Study the drawing (mm; zero at the part's minimum x, y, z) and answer. A direction names the side the tool comes from. Round coordinates to 2 decimals unless told otherwise and drop trailing zeros. Write each loop counter-clockwise with the first axis right and the second up, starting at its lowest first coordinate (ties: lowest second). Pieces come first, ordered by that corner, then holes. Notation, with made-up numbers: (-35.75, 74) - (-18.75, 74) arc R30 ccw to (-18.75, 107) - close; hole circle Ø3 at (79, 56.25). An arc over 180 degrees is marked (long way). Return JSON: item names as keys, results as strings. Group by question number.
(1) Find the intervals of material crossed by line 1 along Z through (x, y) = (1.75, 16); line 2 along Y through (x, z) = (15, 25), in increasing order. Write a range as [from, to].
(2) Determine the mould class of the marked faces 3, 4 and 5 for opening direction Z: +Z half, -Z half, draft (parallel to the pull), parting line (faces both ways), or undercut.
(3) Section A-A, the plane y = 11 is taken. Write down the section's boundary in (x, z), then the cut area to 3 significant figures.
(4) Each of these flat-tipped pins is pushed along its axis until it touches: pin 1 (12 mm diameter, centred on x = 20, y = 9, fed in from +Z); pin 2 (1.4 mm diameter, centred on x = 24, z = 18, fed in from +Y). Where does it stop, or does it pass through?
(5) Section C-C, the plane z = 18 is taken. Write down the section's boundary in (x, y), then the cut area to 3 significant figures.
(6) Which of the six approach directions +Z, -Z, +X, -X, +Y, -Y give full straight-line access (tool end or side, diameter ignored) to the marked faces 1 and 2?
(7) Section D-D, the plane y = 29 is taken. Write down the section's boundary in (x, z), then the cut area to 3 significant figures.
(8) Section B-B, the plane x = 15 is taken. Write down the section's boundary in (y, z).
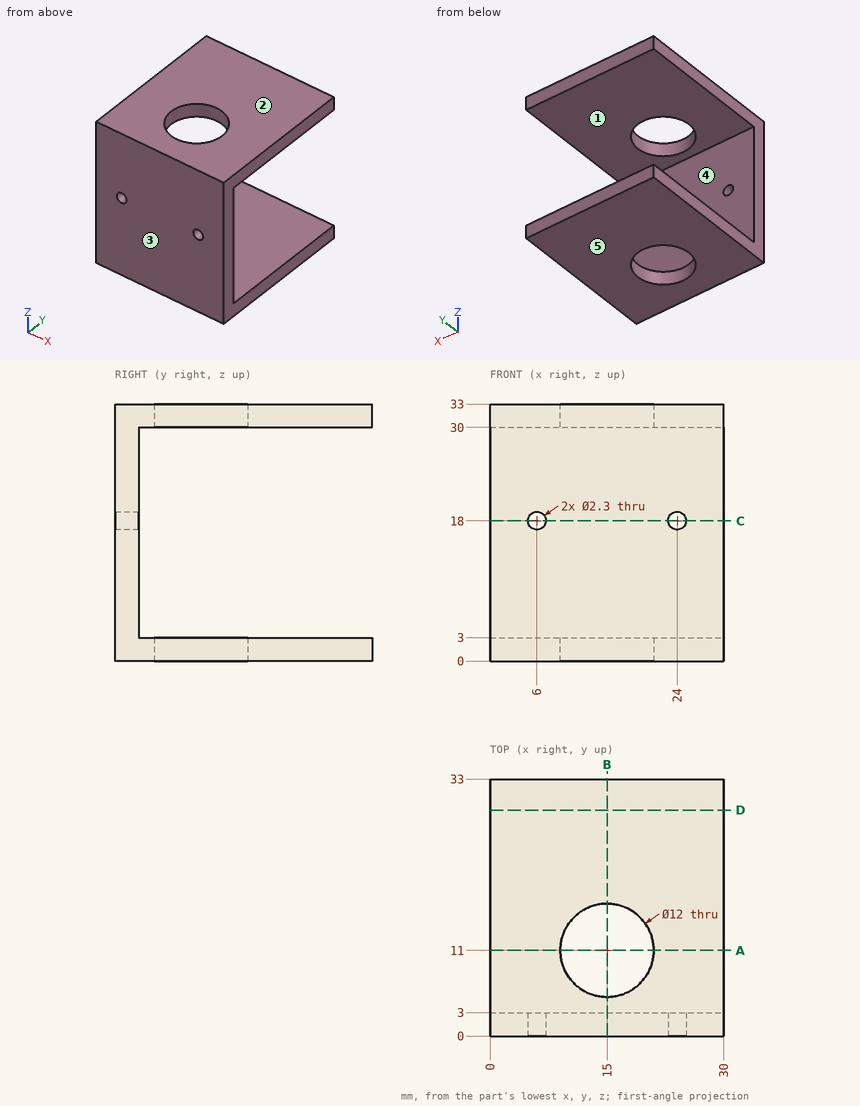
Working result:
{
 "1": {"line 1": "z = [0, 3], [30, 33]", "line 2": "y = [0, 3]"},
 "2": {"face 3": "draft", "face 4": "undercut", "face 5": "-Z half"},
 "3": {"outline": "(0, 0) - (9, 0) - (9, 3) - (0, 3) - close; (0, 30) - (9, 30) - (9, 33) - (0, 33) - close; (21, 0) - (30, 0) - (30, 3) - (21, 3) - close; (21, 30) - (30, 30) - (30, 33) - (21, 33) - close", "area": "108 mm^2"},
 "4": {"pin 1": "stops at z = 33", "pin 2": "passes through"},
 "5": {"outline": "(0, 0) - (4.85, 0) - (4.85, 3) - (0, 3) - close; (7.15, 0) - (22.85, 0) - (22.85, 3) - (7.15, 3) - close; (25.15, 0) - (30, 0) - (30, 3) - (25.15, 3) - close", "area": "76.2 mm^2"},
 "6": {"face 1": "+X, -X, +Y", "face 2": "+Z, +X, -X, +Y, -Y"},
 "7": {"outline": "(0, 0) - (30, 0) - (30, 3) - (0, 3) - close; (0, 30) - (30, 30) - (30, 33) - (0, 33) - close", "area": "180 mm^2"},
 "8": {"outline": "(0, 0) - (5, 0) - (5, 3) - (3, 3) - (3, 30) - (5, 30) - (5, 33) - (0, 33) - close; (17, 0) - (33, 0) - (33, 3) - (17, 3) - close; (17, 30) - (33, 30) - (33, 33) - (17, 33) - close"}
}
